Could you check a few things on this model? Use its own coordinates, in mm. Coordinates: 2 decimals unless noted, no trailing zeros. Write each loop counter-clockwise with the first axis right and the second up, starting at its lowest first coordinate (ties: lowest second). Pieces come first, ordered by that corner, then holes.
Autodesk Inventor part; units mm, degrees
ref_plane "YZ Plane" through (0, 0, 0) normal (1, 0, 0) x (0, 1, 0)
ref_plane "XZ Plane" through (0, 0, 0) normal (0, 1, 0) x (-1, 0, 0)
ref_plane "XY Plane" through (0, 0, 0) normal (0, 0, 1) x (1, 0, 0)
sketch "Skizze1" plane through (0, 0, 0) normal (0, 1, 0) x (-1, 0, 0)
  line L0 (15, -7.5) -> (-15, -7.5)
  line L1 (-15, -7.5) -> (-15, 7.5)
  line L2 (-15, 7.5) -> (15, 7.5)
  line L3 (15, 7.5) -> (15, -7.5)
  line L4 (15, -7.5) -> (-15, 7.5) construction
  line L5 (-15, -7.5) -> (15, 7.5) construction
  point P0 (0, 0)
  dimension "d0" = 15
  dimension "d1" = 30
extrude "Extrusion1" add sketch "Skizze1" along normal blind 15
sketch "Skizze2" plane through (15, 0, 7.5) normal (1, 0, 0) x (0, 0, -1)
  circle A0 centre (7.5, 7.5) radius 4
  line L0 (0, 0) -> (0, 15)
  point P0 (7.5, 0)
  dimension "d4" = 7.5
  dimension "d5" = 8
  dimension "d47" = 7.5
hole "Bohrung1" at (15, 7.5, 0) direction (-1, 0, 0) diameter 4.917 depth 20 tip angle 118
sketch "Skizze4" plane through (-15, 0, 7.5) normal (0, 0, 1) x (1, 0, 0)
  circle A0 centre (7.5, 7.5) radius 2.1663
  line L0 (30, 0) -> (0, 0)
  line L1 (0, 0) -> (0, 15)
  circle A1 centre (22, 15) radius 3.1386
  line L2 (30, 0) -> (30, 15)
  point P0 (15, 0)
  dimension "d27" = 7.5
  dimension "d28" = 7.5
  dimension "d29" = 15
  dimension "d30" = 8
hole "Bohrung3" at (-7.5, 7.5, 7.5) direction (0, 0, -1) diameter 4.917 depth 15 tip angle 118
properties part number "alublock" material "Kupfer"
1. I want a section at B-B on y = 7.5. Please give me the cut outline in (x, z).
Verdict:
outline: (-15, -7.5) - (-9.96, -7.5) - (-9.96, 7.5) - (-15, 7.5) - close; (-5.04, -7.5) - (15, -7.5) - (15, -2.46) - (-5, -2.46) - (-5.04, -2.39) - close; (-5.04, 2.39) - (-5, 2.46) - (15, 2.46) - (15, 7.5) - (-5.04, 7.5) - close
2. For pin 1 (1.5 mm diameter, centred on y = 8, z = -1.5, fed in from +X), with a flat end and sliding along its axis, tell me the tip position at first contact or that it passes through.
Verdict:
pin 1: stops at x = -5.08
3. I want a section at C-C on x = -1. Please give me the cut outline in (y, z).
Verdict:
outline: (0, -7.5) - (15, -7.5) - (15, 7.5) - (0, 7.5) - close; hole circle Ø4.92 at (7.5, 0)
4. If we mould it in two halves opening along Z, with no side actions, what happens to faces 1 (the face through (-5.467, 9.166, 0.219)), 2 (the face through (0, 15, 0)), 3 (the face through (0, 7, -7.5)), 4 (the face through (4.9, 9.7, -1.1))? For each: pulls with the +Z half, pulls with the -Z half, needs draft (parallel to the pull), parting line crosses it, or undercut.
Verdict:
face 1: undercut
face 2: needs draft
face 3: pulls with the -Z half
face 4: undercut
5. Please list where these lines run through material, in increasing order: line 1 along Y through (x, z) = (4.25, 0); line 2 along Z through (x, y) = (7.5, 7.5); line 3 along X through (y, z) = (7.5, 0).
Verdict:
line 1: y = 0 to 5.04, 9.96 to 15
line 2: z = -7.5 to -2.46, 2.46 to 7.5
line 3: x = -15 to -9.96
6. I want a section at D-D on y = 6. Give the number of separate pieces and of enclosed holes in the cut face, plus the area to 3 significant figures.
Verdict:
separate pieces: 3
enclosed holes: 0
area: 312 mm2
7. I want a section at A-A on x = -7.5. Please give me the cut outline in (y, z).
Verdict:
outline: (0, -7.5) - (5.04, -7.5) - (5.04, 7.5) - (0, 7.5) - close; (9.96, -7.5) - (15, -7.5) - (15, 7.5) - (9.96, 7.5) - close
